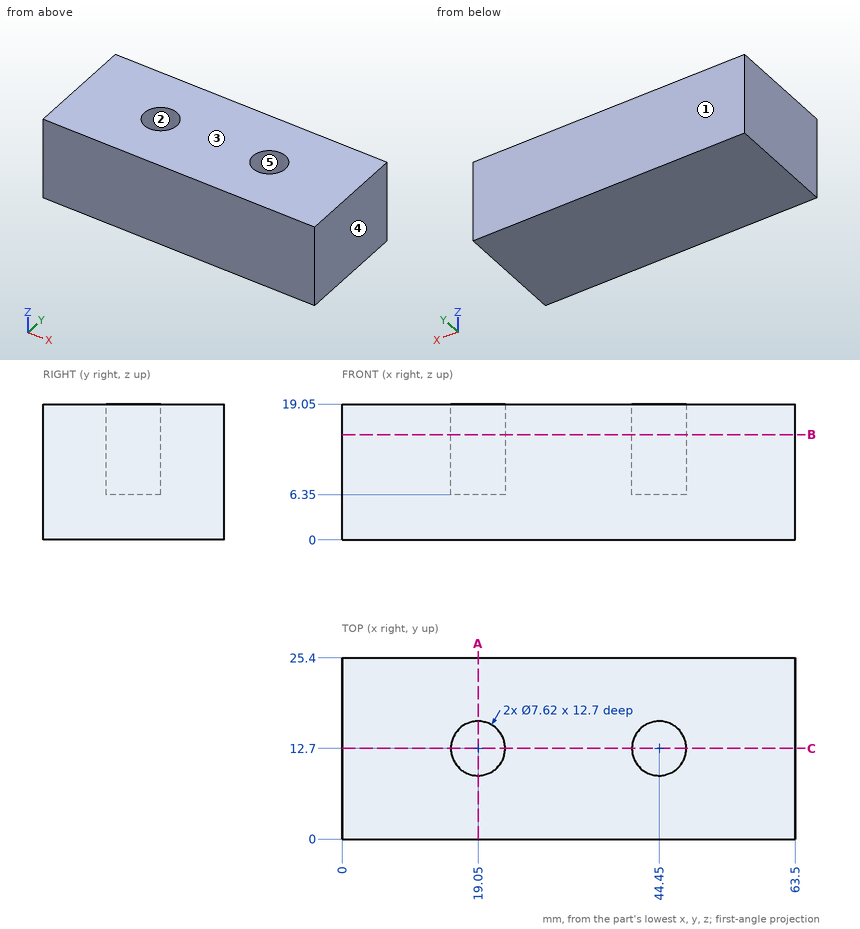
Design review of the part shown in the three views and the two pictorial views. Dimensions are in mm from the part's minimum x, y and z. A direction names the side the tool comes from. Give positions to 0.01 mm unless a question says otherwise; leave off trailing zeros. Write each loop counter-clockwise with the first axis right and the second up, starting at its lowest first coordinate (ties: lowest second). Pieces come first, ordered by that corner, then holes. Notation, with made-up numbers: M 1,23.5 L 33,23.5 A24 ccw 33,52.5 Z; hole C 13.25,-32.75 d10. An arc over 180 degrees is marked long. One line per question, with ' | ' between items. Start each with the question number.
Item 1: We need section A-A on x = 19.05. Write out the cut boundary in (y, z), plus the area to 3 significant figures.
Item 2: We need section B-B on z = 14.75. Write out the cut boundary in (x, y), plus the area to 3 significant figures.
Item 3: For the marked faces 1 and 2, list the 3-axis set-ups (+Z, -Z, +X, -X, +Y, -Y) from which the entire face can be reached by the end or side of a thin tool; tool diameter is ignored.
Item 4: Wall thickness on line 1 (Y direction, x = 19.05, z = 10.5); line 2 (X direction, y = 12, z = 6.5): over which ranges is each line inside the solid? List them lowest first. Write a range as from..to.
Item 5: We need section C-C on y = 12.7. Write out the cut boundary in (x, z), plus the area to 3 significant figures.
Item 6: For pin 1 (7 mm diameter, centred on x = 44.45, y = 12.7, fed in from +Z), flat-tipped, find the tip position at first contact; note if it passes through.
Item 7: Draft analysis for pull direction X (two halves, no side actions). For the marked faces 3, 4 and 5, state which applies: released by +X, released by -X, zero draft, split by the parting line, or undercut.
Results found:
1) outline: M 0,0 L 25.4,0 L 25.4,19.05 L 16.51,19.05 L 16.51,6.35 L 8.89,6.35 L 8.89,19.05 L 0,19.05 Z | area: 387 mm2
2) outline: M 0,0 L 63.5,0 L 63.5,25.4 L 0,25.4 Z; hole C 19.05,12.7 d7.62; hole C 44.45,12.7 d7.62 | area: 1,520 mm2
3) face 1: +Z, -Z, +X, -X, +Y | face 2: +Z
4) line 1: y = 0..8.89, 16.51..25.4 | line 2: x = 0..15.3, 22.8..40.7, 48.2..63.5
5) outline: M 0,0 L 63.5,0 L 63.5,19.05 L 48.26,19.05 L 48.26,6.35 L 40.64,6.35 L 40.64,19.05 L 22.86,19.05 L 22.86,6.35 L 15.24,6.35 L 15.24,19.05 L 0,19.05 Z | area: 1,020 mm2
6) pin 1: stops at z = 6.35
7) face 3: zero draft | face 4: released by +X | face 5: undercut
